Study the drawing (mm; zero at the part's minimum x, y, z) and answer. A direction names the side the tool comes from. Round coordinates to 2 decimals unless told otherwise and drop trailing zeros. Loops run counter-clockwise (first coordinate to the right, second up) from the corner with the lowest first, then second, coordinate; pieces in that order, holes last. Notation, with made-up numbers: M -38,82.5 L 13,82.5 A17 cw 13,93.5 Z; hole C 28.5,84.5 d6. An arc over 180 degrees is marked long. Write each question's results on one line, items separated by ' | '.
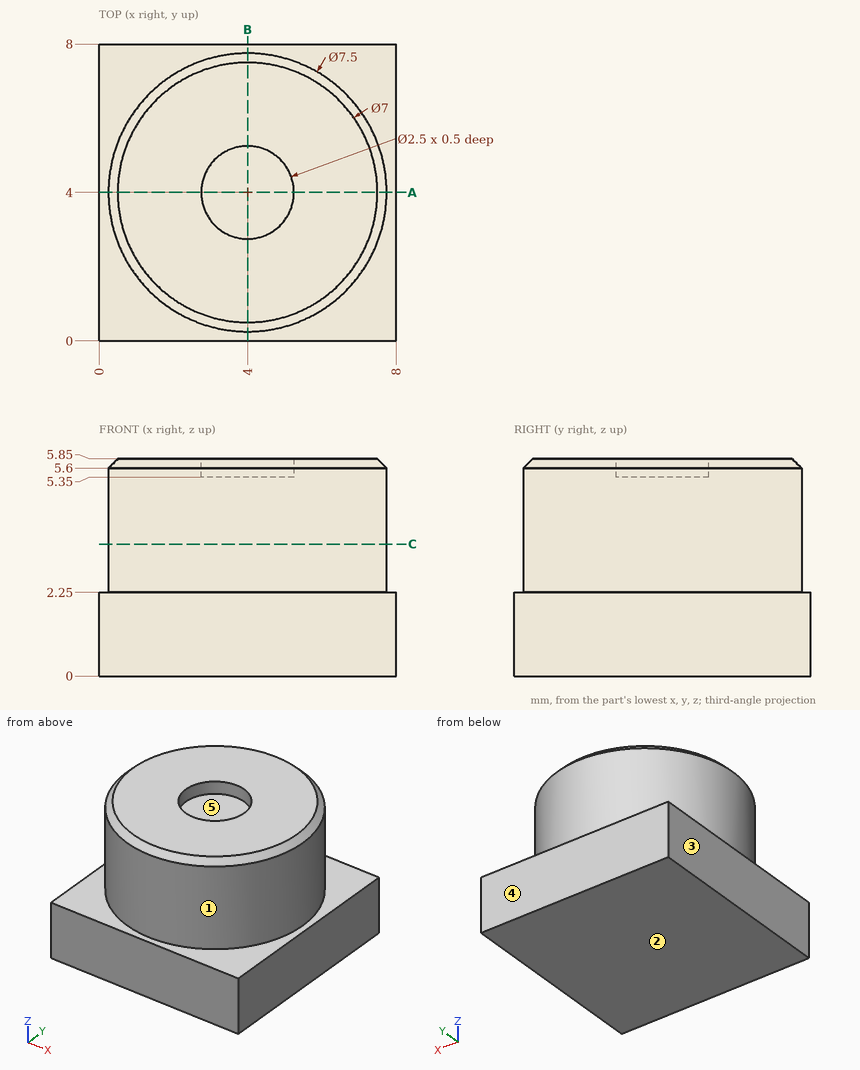
Item 1: The mould has two halves that part along X. Classify the marked faces 3, 4 and 5: pulls with the +X half, pulls with the -X half, needs draft (parallel to the pull), parting line crosses it, or undercut.
Outcome:
face 3: pulls with the -X half | face 4: needs draft | face 5: undercut
Item 2: The part is cut by section C-C (z = 3.55). Determine the outline of the cut face in (x, y), plus the area to 3 significant figures.
Outcome:
outline: C 4,4 d7.5 | area: 44.2 mm2
Item 3: For the marked faces 1 and 2, determine the directions among +Z, -Z, +X, -X, +Y, -Y from which every point of the face is accessible in a straight line to the end or side of a thin tool.
Outcome:
face 1: +Z | face 2: -Z, +X, -X, +Y, -Y
Item 4: Flat-ended cylindrical pins translate along their axes: pin 1 (1 mm diameter, centred on y = 6.5, z = 4.5, fed in from +X); pin 2 (2 mm diameter, centred on y = 4.5, z = 4.5, fed in from -X). Find the tip coordinate at first contact, or state that the pin passes through.
Outcome:
pin 1: stops at x = 7.17 | pin 2: stops at x = 0.25
Item 5: The part is cut by section A-A (y = 4). Determine the outline of the cut face in (x, z).
Outcome:
outline: M 0,0 L 8,0 L 8,2.25 L 7.75,2.25 L 7.75,5.6 L 7.5,5.85 L 5.25,5.85 L 5.25,5.35 L 2.75,5.35 L 2.75,5.85 L 0.5,5.85 L 0.25,5.6 L 0.25,2.25 L 0,2.25 Z
Item 6: Straight lines are drawn through the part: line 1 (Y direction, x = 4, z = 5.55); line 2 (Y direction, x = 4, z = 5.7); line 3 (Z direction, x = 4.25, y = 3.75). For each, find the intervals that lie inside material, in ascending order.
Outcome:
line 1: y = 0.25 to 2.75, 5.25 to 7.75 | line 2: y = 0.35 to 2.75, 5.25 to 7.65 | line 3: z = 0 to 5.35
